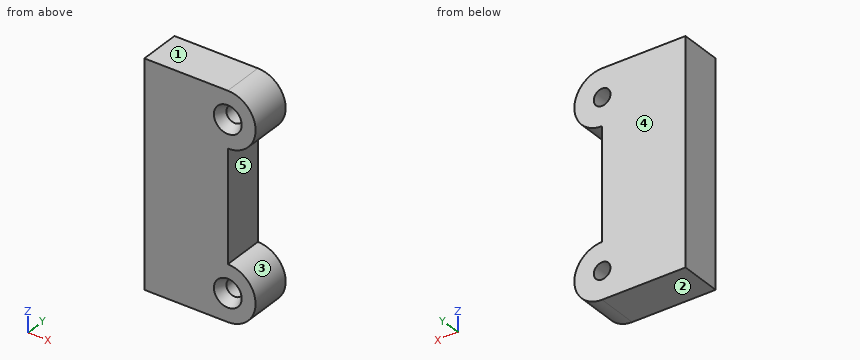
from build123d import *

# Parameters (mm, degrees)
F1_DEPTH       = 9.525
F3_D           = 3.81
F3_CSINK_D     = 6.35
F3_CSINK_ANGLE = 60


with BuildPart() as f1:
    # F0 (on Front) → F1 (new body)
    with BuildSketch(Plane.XZ):
        with BuildLine():
            Line((0, 50.8), (0, 0))
            Line((0, 0), (19.05, 0))
            ThreePointArc((19.05, 0), (25.4, 6.35), (19.05, 12.7))
            Line((19.05, 12.7), (19.05, 38.1))
            ThreePointArc((19.05, 38.1), (25.4, 44.45), (19.05, 50.8))
            Line((19.05, 50.8), (0, 50.8))
        make_face()
    extrude(amount=F1_DEPTH)

    # F3 (through all)
    with Locations(Plane.XZ.offset(9.525)):
        with Locations((19.05, 44.45), (19.05, 6.35)):
            CounterSinkHole(F3_D / 2, F3_CSINK_D / 2, counter_sink_angle=F3_CSINK_ANGLE)


solid = f1.part
Check sheet for the modelled part. Datum: model origin and axes. Units: mm. Face numbers are marked on the shaded views. A direction names the side the tool comes from. Round coordinates to 2 decimals unless told otherwise and drop trailing zeros. Order: outer loops, then holes, each group sorted by start corner. A loop starts at its lowest first (then second) coordinate and runs counter-clockwise, first axis right, second up.
(1) Scan lines: probe 1 along X at (y, z) = (-1.75, 44.45) (3 decimals); probe 2 along X at (y, z) = (-5.75, 6.5); probe 3 along X at (y, z) = (-1, 24). Record each from-to range of solid material in increasing order.
(2) Cross-section at C-C, the plane z = 28. Enter the section's corners in (x, y) (3 decimals), and give its area (3 significant figures).
(3) Cross-section at D-D, the plane y = -9. Enter the section's corners in (x, z).
(4) Cross-section at A-A, the plane z = 6.35. Enter the section's corners in (x, y) (3 decimals).
(5) Access from +Z, -Z, +X, -X, +Y, -Y to the whole of each face (thin tool, end or side, straight path). Record for the marked faces 4 and 5.
(6) Draft check along Z on the marked faces 1, 2 and 3. Enter one of: pulls with the +Z half, pulls with the -Z half, needs draft (parallel to the pull), parting line crosses it, or undercut.
(7) Go/stop test with a flat-tipped pin: P1, Ø5, axis at y = -6.5, z = 31.5, coming from the +X side. Record where the tip stops, or that it passes through.
(8) Cross-section at B-B, the plane y = -1.75. Enter the section's corners in (x, z) (3 decimals).
Check sheet entries:
1. probe 1: x = 0 to 17.145, 20.955 to 25.4
1. probe 2: x = 0 to 17.15, 20.95 to 25.4
1. probe 3: x = 0 to 19.05
2. outline: (0, -9.525) - (19.05, -9.525) - (19.05, 0) - (0, 0) - close
2. area: 181 mm2
3. outline: (0, 0) - (19.05, 0) arc R6.35 ccw to (19.05, 12.7) - (19.05, 38.1) arc R6.35 ccw to (19.05, 50.8) - (0, 50.8) - close; hole circle Ø5.74 at (19.05, 6.35); hole circle Ø5.74 at (19.05, 44.45)
4. outline: (0, -9.525) - (15.875, -9.525) - (17.145, -7.325) - (17.145, 0) - (0, 0) - close; (20.955, -7.325) - (22.225, -9.525) - (25.4, -9.525) - (25.4, 0) - (20.955, 0) - close
5. face 4: +Z, -Z, +X, -X, +Y
5. face 5: +X, +Y, -Y
6. face 1: pulls with the +Z half
6. face 2: pulls with the -Z half
6. face 3: undercut
7. P1: stops at x = 19.05
8. outline: (0, 0) - (19.05, 0) arc R6.35 ccw to (19.05, 12.7) - (19.05, 38.1) arc R6.35 ccw to (19.05, 50.8) - (0, 50.8) - close; hole circle Ø3.81 at (19.05, 6.35); hole circle Ø3.81 at (19.05, 44.45)
